For this review, take the finished solid that the model builds, in its own axes (mm). Face numbers are marked on the shaded views. A direction names the side the tool comes from. Give positions to 0.01 mm unless a question says otherwise; leave off trailing zeros. Loops run counter-clockwise (first coordinate to the right, second up) from the corner with the lowest first, then second, coordinate; pieces in that order, holes last. Notation, with made-up numbers: (83, 30.5) - (87, 30.5) arc R22 ccw to (87, 53.5) - close; hole circle Ø4 at (6, 15.25). An arc over 180 degrees is marked (long way). Answer in a Markdown table with one row per item.
Autodesk Inventor part; units mm, degrees
ref_plane "YZ Plane" through (0, 0, 0) normal (1, 0, 0) x (0, 1, 0)
ref_plane "XZ Plane" through (0, 0, 0) normal (0, 1, 0) x (-1, 0, 0)
ref_plane "XY Plane" through (0, 0, 0) normal (0, 0, 1) x (1, 0, 0)
sketch "Sketch1" plane through (0, 0, 0) normal (0, 0, 1) x (1, 0, 0)
  line L0 (0, 0) -> (0, 5)
  line L1 (0, 5) -> (0, 30)
  line L2 (0, 30) -> (0, 35)
  line L3 (0, 35) -> (10, 35)
  line L4 (10, 35) -> (10, 0)
  line L5 (10, 0) -> (0, 0)
  line L6 (0, 35) -> (5, 35)
  line L7 (5, 35) -> (5, 0)
  circle A0 centre (5, 30) radius 1.5
  circle A1 centre (5, 5) radius 1.5
  line L8 (5, 17.5) -> (10, 17.5)
  line L9 (10, 17.5) -> (16, 17.5)
  line L10 (16, 17.5) -> (16, 12.5)
  line L11 (16, 17.5) -> (16, 22.5)
  line L12 (16, 22.5) -> (10, 35)
  line L13 (16, 12.5) -> (10, 0)
  dimension "d0" = 5
  dimension "d1" = 25
  dimension "d2" = 5
  dimension "d3" = 10
  dimension "d4" = 5
  dimension "d5" = 3
  dimension "d6" = 3
  dimension "d7" = 6
  dimension "d8" = 5
  dimension "d9" = 5
extrude "Extrusion1" add sketch "Sketch1" along normal blind 6 contours L0 L1 L2 L3 L7 A0 A1 L5 | L7 A1 L8 L4 L5 | L4 L9 L10 L13 | L8 L7 A0 L3 L4 | L4 L12 L11 L9
sketch "Sketch2" plane through (0, 0, 0) normal (0, 0, -1) x (-1, 0, 0)
  line L0 (0, 35) -> (0, 0)
  line L1 (-10, 35) -> (0, 35)
  line L2 (-16, 22.5) -> (-10, 35)
  line L3 (-16, 12.5) -> (-16, 22.5)
  line L4 (-10, 0) -> (-16, 12.5)
  line L5 (0, 0) -> (-10, 0)
  circle A0 centre (-5, 30) radius 1.5
  circle A1 centre (-5, 5) radius 1.5
  line L6 (-10, 0) -> (-16, 12.5)
  line L7 (-10, 35) -> (-10, 0)
  line L8 (-10, 0) -> (-16, 12.5)
  line L9 (-16, 12.5) -> (-16, 22.5)
  line L10 (-10, 35) -> (-16, 22.5)
  line L11 (-10.2, 34.5833) -> (-10.2, 0.4167)
  point P0 (-10.2, 0.4167)
  dimension "d54" = 0.2
extrude "Extrusion2" add sketch "Sketch2" along normal blind 8.5 contours L11 L4 L3 L2
sketch "Sketch3" plane through (0, 0, 6) normal (0, 0, 1) x (1, 0, 0)
  line L0 (0, 35) -> (0, 0)
  line L1 (0, 0) -> (10, 0)
  line L2 (10, 0) -> (16, 12.5)
  line L3 (16, 12.5) -> (16, 22.5)
  line L4 (16, 22.5) -> (10, 35)
  line L5 (10, 35) -> (0, 35)
  circle A0 centre (5, 30) radius 1.5
  circle A1 centre (5, 5) radius 1.5
  circle A2 centre (5, 30) radius 3.25
  circle A3 centre (5, 5) radius 3.25
  dimension "d14" = 6.5
  dimension "d17" = 6.5
extrude "Extrusion3" cut sketch "Sketch3" against normal blind 3 contours A0 | A2 | A3
sketch "Sketch4" plane through (0, 0, -8.5) normal (0, 0, -1) x (-1, 0, 0)
  line L0 (-10.2, 34.5833) -> (-16, 22.5)
  line L1 (-16, 22.5) -> (-16, 12.5)
  line L2 (-16, 12.5) -> (-10.2, 0.4167)
  line L3 (0, 0) -> (-10, 0)
  line L4 (0, 35) -> (0, 0)
  line L5 (-10, 35) -> (0, 35)
  circle A0 centre (-5, 30) radius 1.5
  circle A1 centre (-5, 5) radius 1.5
  line L6 (-15.8046, 22.9071) -> (-13.1, 21.609)
  line L7 (-15.8046, 12.0929) -> (-13.1, 13.391)
  circle A2 centre (-13.1, 13.391) radius 1
  circle A3 centre (-13.1, 21.609) radius 1
  line L8 (-10.2, 34.5833) -> (-10.2, 0.4167)
  line L9 (-10, 0) -> (-10.2, 0.4167)
  line L10 (-10.2, 34.5833) -> (-10, 35)
  line L11 (-10.2, 0.4167) -> (-10.2, 34.5833)
  dimension "d39" = 3
  dimension "d41" = 90
  dimension "d42" = 3
  dimension "d43" = 90
  dimension "d45" = 2.9
  dimension "d46" = 2
  dimension "d47" = 2
  dimension "d52" = 8.2179
  dimension "d55" = 2.9
  dimension "d56" = 0.2
  dimension "d57" = 6
extrude "Extrusion4" cut sketch "Sketch4" against normal blind 8 contours A3 | A2
equation "\"d2\" = d0"
equation "\"d4\" = 0.5 * d3"
equation "\"d9\" = d8"
equation "\"d39\" = 0.5 * d36"
equation "\"d42\" = d39"
equation "\"d45\" = d55"
equation "\"d55\" = -0.5 * d56 + 0.5 * d57"
properties part number "Clamp"
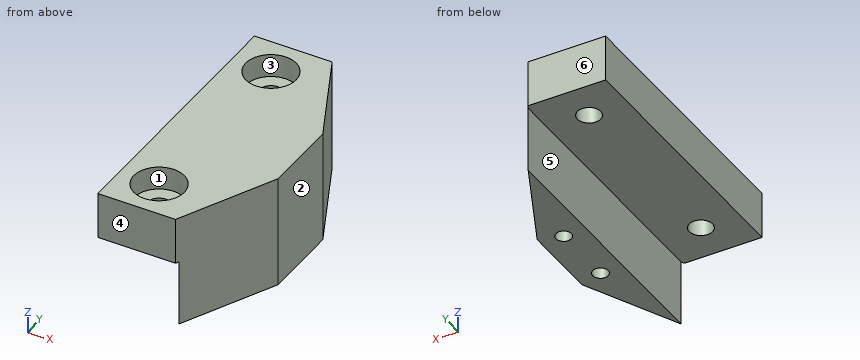
1. Wall thickness on line 1 (Y direction, x = 5, z = 2.4); line 2 (Y direction, x = 13.1, z = -2); line 3 (Z direction, x = 2, y = 1): over which ranges is each line inside the solid? List them lowest first. Write a range as [from, to].
Values:
| item | result |
|---|---|
| line 1 | y = [0, 3.5], [6.5, 28.5], [31.5, 35] |
| line 2 | y = [6.46, 12.39], [14.39, 20.61], [22.61, 28.54] |
| line 3 | z = [0, 6] |
2. We need section A-A, the plane y = 5. Give the boundary of the cut face in (x, z).
Values:
| item | result |
|---|---|
| outline | (0, 0) - (3.5, 0) - (3.5, 3) - (1.75, 3) - (1.75, 6) - (0, 6) - close; (6.5, 0) - (10.2, 0) - (10.2, -8.5) - (12.4, -8.5) - (12.4, 6) - (8.25, 6) - (8.25, 3) - (6.5, 3) - close |
3. Mouldability with a two-part tool opening along Y and no side actions: class the marked faces 1, 2, 3 and 4 as released by +Y, released by -Y, zero draft, split by the parting line, or undercut.
Values:
| item | result |
|---|---|
| face 1 | undercut |
| face 2 | zero draft |
| face 3 | undercut |
| face 4 | released by -Y |
4. For the marked faces 5 and 6, list the 3-axis set-ups (+Z, -Z, +X, -X, +Y, -Y) from which the entire face can be reached by the end or side of a thin tool; tool diameter is ignored.
Values:
| item | result |
|---|---|
| face 5 | -Z, -X, +Y, -Y |
| face 6 | +Z, -Z, +X, -X, +Y |
5. Clearance check with flat-ended pins moving along their axes: pin 1 (6 mm diameter, centred on x = 5, y = 5, fed in from +Z); pin 2 (4 mm diameter, centred on y = 22.5, z = -5, fed in from -X); pin 3 (7.5 mm diameter, centred on x = 5, y = 30, fed in from -Z). State where each tip first meets the part, or that it passes through.
Values:
| item | result |
|---|---|
| pin 1 | stops at z = 3 |
| pin 2 | stops at x = 10.2 |
| pin 3 | stops at z = 0 |
6. We need section C-C, the plane z = 4.5. Give the boundary of the cut face in (x, y).
Values:
| item | result |
|---|---|
| outline | (0, 0) - (10, 0) - (16, 12.5) - (16, 22.5) - (10, 35) - (0, 35) - close; hole circle Ø6.5 at (5, 5); hole circle Ø6.5 at (5, 30) |
7. We need section D-D, the plane y = 18. Give the boundary of the cut face in (x, z), and give its area (3 significant figures).
Values:
| item | result |
|---|---|
| outline | (0, 0) - (10.2, 0) - (10.2, -8.5) - (16, -8.5) - (16, 6) - (0, 6) - close |
| area | 145 mm^2 |
8. We need section B-B, the plane x = 5. Give the boundary of the cut face in (y, z).
Values:
| item | result |
|---|---|
| outline | (0, 0) - (3.5, 0) - (3.5, 3) - (1.75, 3) - (1.75, 6) - (0, 6) - close; (6.5, 0) - (28.5, 0) - (28.5, 3) - (26.75, 3) - (26.75, 6) - (8.25, 6) - (8.25, 3) - (6.5, 3) - close; (31.5, 0) - (35, 0) - (35, 6) - (33.25, 6) - (33.25, 3) - (31.5, 3) - close |
